from build123d import *

# Parameters (mm, degrees)
BOSS_EXTRUDE1_DEPTH   = 40
BODY_MOVE_COPY1_ANGLE = 20
BOSS_EXTRUDE2_DEPTH   = 2
BOSS_EXTRUDE3_DEPTH   = 12
SKETCH4_R             = 2.5
CUT_EXTRUDE2_DEPTH    = 8
FILLET1_R             = 2
SKETCH10_W            = 4.9
SKETCH10_H            = 3
SKETCH10_W_2          = 5.1
SKETCH10_W_3          = 5
CUT_EXTRUDE4_DEPTH    = 2
FILLET2_R             = 0.5


with BuildPart() as part:
    # Sketch2 → Boss-Extrude1 (new body)
    with BuildSketch(Plane.XY):
        Polygon((90, 0), (105, 0), (105, 3), (93, 30), (90, 30), align=None)
    extrude(amount=BOSS_EXTRUDE1_DEPTH)


with BuildPart() as part_1:
    # Body-Move_Copy1: moved
    add(part.part.rotate(Axis((95, 0, 20), (0, -1, 0)), BODY_MOVE_COPY1_ANGLE))


with BuildPart() as part_2:
    # Body-Move_Copy2: moved
    add(part_1.part.moved(Location((-2, 0, -25))))

    # Sketch1 → Boss-Extrude2 (add)
    with BuildSketch(Plane(origin=(0, 0, 0), x_dir=(1, 0, 0), z_dir=(0, 1, 0))):
        Polygon((0, 49), (0, 0), (77, 0), (83.495200367, -6.495200367), (88.832123786, 8.167876214), (87, 10), (87, 49), align=None)
    extrude(amount=BOSS_EXTRUDE2_DEPTH)

    # Sketch1_4 → Boss-Extrude3 (add)
    with BuildSketch(Plane(origin=(0, 0, 0), x_dir=(1, 0, 0), z_dir=(0, 1, 0))):
        Polygon((8, 43), (8, 46), (39.9, 46), (39.9, 43), (44.9, 43), (44.9, 46), (79, 46), (79, 43), (83.9, 43), (83.9, 6), (79, 6), (79, 3), (44.9, 3), (44.9, 6), (39.9, 6), (39.9, 3), (8, 3), (8, 6), (2.9, 6), (2.9, 13), (0, 13), (0, 0), (77, 0), (87, 0), (87, 10), (87, 49), (0, 49), (0, 36), (2.9, 36), (2.9, 43), align=None)
    extrude(amount=BOSS_EXTRUDE3_DEPTH)

    # Sketch4 → Cut-Extrude2 (cut)
    with BuildSketch(Plane(origin=(76.126595154, 36.005435759, 27.707814672), x_dir=(0.29946549765090347, 0.09724282163216282, -0.9491386881576961), z_dir=(0.8587019690275818, 0.40613846605344794, 0.3125419568312492))):
        with Locations(Location((42.744832372, -18.834040509, 0), (0, 0, 92.300030603))):
            Circle(SKETCH4_R)
        with Locations(Location((41.048584848, -34.683530859, 0), (0, 0, 92.300030603))):
            Circle(SKETCH4_R)
    extrude(amount=-CUT_EXTRUDE2_DEPTH, mode=Mode.SUBTRACT)

    # Fillet1
    fillet1_edges = [part_2.edges().sort_by_distance(p)[0] for p in [
        (82.870672961, 30, 12.596781914),
        (96.551478694, 30, -24.990922917),
    ]]
    fillet(fillet1_edges, radius=FILLET1_R)

    # Sketch10 → Cut-Extrude4 (cut)
    with BuildSketch(Plane(origin=(0, 12, 0), x_dir=(1, 0, 0), z_dir=(0, 1, 0))):
        with Locations((81.45, 4.5)):
            Rectangle(SKETCH10_W, SKETCH10_H)
        with Locations((42.45, 4.5)):
            Rectangle(SKETCH10_W_2, SKETCH10_H)
        with Locations((42.4, 44.5)):
            Rectangle(SKETCH10_W_3, SKETCH10_H)
        with Locations((81.45, 44.5)):
            Rectangle(SKETCH10_W, SKETCH10_H)
        with Locations((5.45, 44.5)):
            Rectangle(SKETCH10_W_2, SKETCH10_H)
        with Locations((5.45, 4.5)):
            Rectangle(SKETCH10_W_2, SKETCH10_H)
    extrude(amount=-CUT_EXTRUDE4_DEPTH, mode=Mode.SUBTRACT)

    # Fillet2
    fillet2_edges = [part_2.edges().sort_by_distance(p)[0] for p in [
        (88.301536896, 30, -6.710100717),
        (81.46113403, 14, 12.083751699),
        (95.141939763, 14, -25.503953132),
        (81.661484791, 29.414213562, 11.533292506),
        (94.941589001, 29.414213562, -24.95349394),
        (87, 6, -49),
        (0, 6, -49),
        (0, 6, 0),
        (2.9, 12, -41),
        (43.4, 12, -46),
        (83.9, 12, -24.5),
        (2.9, 12, -8),
        (43.4, 12, -3),
    ]]
    fillet(fillet2_edges, radius=FILLET2_R)


solid = part_2.part
Read the model definition and answer for the solid it produces. Units are mm, in the model's axes. A direction names the side the tool comes from. Give positions to 0.01 mm unless a question says otherwise; leave off trailing zeros. Write each loop counter-clockwise with the first axis right and the second up, starting at its lowest first coordinate (ties: lowest second). Pieces come first, ordered by that corner, then holes. Notation, with made-up numbers: (8, 36.25) - (59, 36.25) arc R12 ccw to (59, 58.25) - close; hole circle Ø6 at (11, 5.25). An arc over 180 degrees is marked (long way). Use CSV: the item, a comma, the result in double quotes. Start each with the question number.
(1) Consider line 1 along X through (y, z) = (9, -44); line 2 along Z through (x, y) = (25.5, 7.5); line 3 along X through (y, z) = (5, -4). Determine where each line is inside the solid, lowest interval first.
(2) Find section B-B (x = 12). Give the vertices of the cut face in (y, z), plus the area to 3 significant figures.
(3) Find section A-A (z = -39). Give the vertices of the cut face in (x, y), plus the area to 3 significant figures.
(4) Find section D-D (y = 15). Give the vertices of the cut face in (x, z).
(5) For faces 1 (the flat face through (90, 30, -6)), 2 (the flat face through (82, 2, 2)), 3 (the flat face through (50, 12, -1)), 4 (the flat face through (83.9, 7, -24)), determine the directions among +Z, -Z, +X, -X, +Y, -Y from which every point of the face is accessible in a straight line to the end or side of a thin tool.
(6) Determine the mould class of faces 5 (the flat face through (43, 6, 0)), 6 (the flat face through (39.9, 6, -5)), 7 (the cylindrical face through (88.35, 29.85, -6.42)) for opening direction X: +X half, -X half, draft (parallel to the pull), parting line (faces both ways), or undercut.
(7) Find section C-C (x = 41). Give the vertices of the cut face in (y, z).
(8) Given P1, Ø5, axis at y = 5.5, z = -11, coming from the +X side; P2, Ø1.5, axis at x = 87.5, z = -5.5, coming from the +Y side; P3, Ø2.5, axis at x = 5.5, z = -45, coming from the +Y side, each flat-ended and moving along its own axis, determine where each tip first touches the part or whether it passes through.
Findings below:
1,line 1,"0 to 8, 39.9 to 44.9, 79 to 87"
1,line 2,"-49 to -46, -3 to 0"
1,line 3,"0 to 8, 39.9 to 44.9, 79 to 87, 87.32 to 102.33"
2,outline,"(0, -49) - (12, -49) - (12, -46.5) arc R0.5 ccw to (11.5, -46) - (2, -46) - (2, -3) - (11.5, -3) arc R0.5 ccw to (12, -2.5) - (12, 0) - (0, 0) - close"
2,area,"158 mm2"
3,outline,"(0, 0) - (87, 0) - (87, 12) - (84.4, 12) arc R0.5 ccw to (83.9, 11.5) - (83.9, 2) - (2.9, 2) - (2.9, 11.5) arc R0.5 ccw to (2.4, 12) - (0, 12) - close"
3,area,"234 mm2"
4,outline,"(81.63, 11.61) - (94.97, -25.03) arc R0.5 ccw to (95.61, -25.33) - (104.23, -22.2) - (90.54, 15.39) - (81.93, 12.25) arc R0.5 ccw to start"
5,face 1,"+Z, -Z, +X, -X, +Y"
5,face 2,"-X, +Y"
5,face 3,"-Z, -X, +Y"
5,face 4,"+Y"
6,face 5,"draft"
6,face 6,"undercut"
6,face 7,"-X half"
7,outline,"(0, -49) - (12, -49) - (12, -46.5) arc R0.5 ccw to (11.5, -46) - (10, -46) - (10, -43) - (2, -43) - (2, -6) - (10, -6) - (10, -3) - (11.5, -3) arc R0.5 ccw to (12, -2.5) - (12, 0) - (0, 0) - close"
8,P1,"x = 106.14"
8,P2,"y = 29.99"
8,P3,"y = 11.93"
